Autodesk Inventor part; units mm, degrees
ref_plane "YZ Plane" through (0, 0, 0) normal (1, 0, 0) x (0, 1, 0)
ref_plane "XZ Plane" through (0, 0, 0) normal (0, 1, 0) x (-1, 0, 0)
ref_plane "XY Plane" through (0, 0, 0) normal (0, 0, 1) x (1, 0, 0)
sketch "Sketch1" plane through (0, 0, 0) normal (0, 0, 1) x (1, 0, 0)
  line L0 (-26.797, 26.797) -> (26.797, 26.797)
  line L1 (26.797, 26.797) -> (26.797, -26.797)
  line L2 (26.797, -26.797) -> (-26.797, -26.797)
  line L3 (-26.797, -26.797) -> (-26.797, 26.797)
  point P0 (0, 0)
  point P1 (-26.797, 0)
  point P2 (0, 26.797)
  dimension "d0" = 53.594
  dimension "d1" = 53.594
extrude "Extrusion1" add sketch "Sketch1" along normal blind 38.1
fillet "Fillet1" radius 6.35 2 edges at (-26.797, 26.797, 19.05) (26.797, 26.797, 19.05)
sketch "Sketch3" plane through (0, 0, 38.1) normal (0, 0, 1) x (1, 0, 0)
  arc A0 (26.797, 20.447) -> (20.447, 26.797) centre (20.447, 20.447) ccw
  line L0 (-20.447, 26.797) -> (20.447, 26.797)
  arc A1 (-20.447, 26.797) -> (-26.797, 20.447) centre (-20.447, 20.447) ccw
  line L1 (-26.797, -26.797) -> (-26.797, 20.447)
  line L2 (26.797, -26.797) -> (-26.797, -26.797)
  line L3 (26.797, 20.447) -> (26.797, -26.797)
  arc A2 (-22.5612, -14.4593) -> (-20.447, -26.797) centre (-20.447, -20.447) ccw
  arc A3 (20.447, -26.797) -> (22.5612, -14.4593) centre (20.447, -20.447) ccw
  line L4 (-26.797, -26.797) -> (26.797, -26.797)
  line L5 (-26.797, 0) -> (-26.797, -26.797)
  line L6 (26.797, 0) -> (26.797, -26.797)
  arc A4 (22.5612, -14.4593) -> (-22.5612, -14.4593) centre (0, 0) ccw
  line L7 (-26.797, 0) -> (-26.797, 20.447)
  line L8 (-20.447, 26.797) -> (20.447, 26.797)
  line L9 (26.797, 20.447) -> (26.797, 0)
  arc A5 (-20.447, 26.797) -> (-26.797, 20.447) centre (-20.447, 20.447) ccw
  arc A6 (26.797, 20.447) -> (20.447, 26.797) centre (20.447, 20.447) ccw
  dimension "d9" = 12.7
  dimension "d10" = 12.7
  dimension "d12" = 26.797
extrude "Extrusion2" cut sketch "Sketch3" against normal through all contours L3 A3 A4 | L3 L2 A3 | A4 A2 L1 | A2 L2 L1
fillet "Fillet2" radius 1.5875 2 edges at (22.5612, -14.4593, 19.05) (-22.5612, -14.4593, 19.05)
sketch "Sketch4" plane through (-20.447, 26.797, 0) normal (0, 1, 0) x (1, 0, 0)
  line L0 (0, 0) -> (40.894, 0)
  line L1 (-6.35, -38.1) -> (0, -38.1)
  line L2 (0, -38.1) -> (0, 0)
  line L3 (0, 0) -> (-6.35, 0)
  line L4 (-6.35, 0) -> (-6.35, -38.1)
  line L5 (43.8591, 0) -> (43.8591, -38.1)
  line L6 (40.894, -38.1) -> (47.244, -38.1)
  line L7 (47.244, -38.1) -> (47.244, 0)
  line L8 (47.244, 0) -> (40.894, 0)
  line L9 (40.894, 0) -> (40.894, -38.1)
  line L10 (-2.9651, -38.1) -> (-2.9651, 0)
  circle A0 centre (20.447, -25.4) radius 19.05
  point P0 (20.447, 0)
  point P1 (20.447, -6.35)
  point P2 (20.447, 0)
  dimension "d16" = 38.1
  dimension "d17" = 6.35
extrude "Extrusion3" add sketch "Sketch4" along normal blind 3.175 contours A0
fillet "Fillet3" radius 0.7937 1 edges at (-19.05, 29.972, 25.4)
sketch "Sketch5" plane through (0, 29.972, 25.4) normal (0, 1, 0) x (1, 0, 0)
  circle A0 centre (0, 0) radius 18.2562
  circle A1 centre (0, 0) radius 12.7
  circle A2 centre (0, 0) radius 19.05
  point P0 (0, 25.4)
  dimension "d24" = 6.35
extrude "Extrusion4" add sketch "Sketch5" along normal blind 25.4 contours A1
sketch "Sketch6" plane through (0, 29.972, 25.4) normal (0, 1, 0) x (1, 0, 0)
  circle A0 centre (-14.1881, 8.1915) radius 1.6383
  circle A1 centre (0, -16.383) radius 1.6383
  circle A2 centre (14.1881, 8.1915) radius 1.6383
  point P0 (0, 25.4)
hole "Hole1" at (0, 29.972, 41.783) at (14.1881, 29.972, 17.2085) at (-14.1881, 29.972, 17.2085) direction (0, -1, 0) diameter 3.2766 depth 6.35 tip angle 118
properties part number "Pneumatics_VIAIR_0090_02"
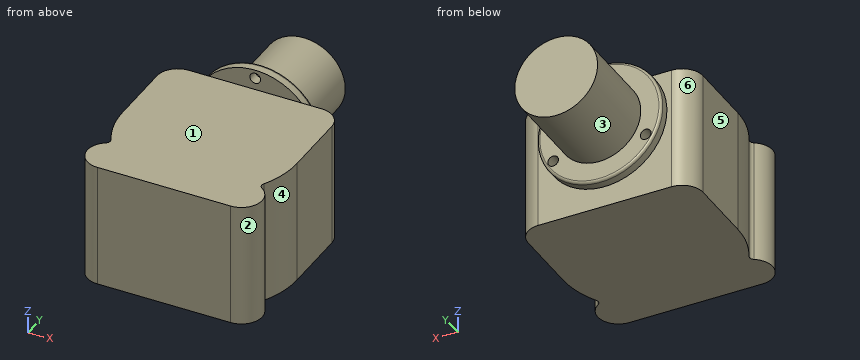
Geometry check sheet. Reference: the model listing, model coordinates, mm. Face numbers are marked on the shaded views. A direction names the side the tool comes from. Round coordinates to 2 decimals unless told otherwise and drop trailing zeros. Order: outer loops, then holes, each group sorted by start corner. A loop starts at its lowest first (then second) coordinate and runs counter-clockwise, first axis right, second up. Notation, with made-up numbers: (-7.5, -36.75) - (43.5, -36.75) arc R28 cw to (43.5, 2.25) - close; hole circle Ø7 at (47, 0). An arc over 180 degrees is marked (long way). One line per question, with ' | ' between items. Start each with the question number.
(1) Sectioned sample at A-A on x = 0. Record the cut outline in (y, z), and give its area (3 significant figures).
(2) Depth check by flat-ended pin: pin 1 Ø2.5 at (x, z) = (14.19, 17.21) entering from +Y; pin 2 Ø3 at (x, y) = (16.5, -7) entering from +Z; pin 3 Ø10 at (y, z) = (38, 36.5) entering from +X. Enter the tip coordinate at first touch or a pass-through.
(3) Sectioned sample at D-D on y = -21. Record the cut outline in (x, z), and give its area (3 significant figures).
(4) Sectioned sample at B-B on y = 35.5. Record the cut outline in (x, z), and give its area (3 significant figures).
(5) Access from +Z, -Z, +X, -X, +Y, -Y to the whole of each face (thin tool, end or side, straight path). Record for the marked faces 1, 2 and 3.
(6) Thickness scan on L1, parallel to Z at x = 0, y = 28.9; L2, parallel to Y at x = -18.5, z = 10.5; L3, parallel to Z at x = -8.5, y = 5.5. Record the ranges inside material, lowest first. Write a range as [from, to].
(7) Sectioned sample at C-C on y = 16.5. Record the cut outline in (x, z).
(8) Release check for a two-part mould opening along Y. For the marked faces 4, 5 and 6 record: released by +Y, released by -Y, zero draft, split by the parting line, or undercut.
Conclusion:
1) outline: (-26.8, 0) - (26.8, 0) - (26.8, 6.35) - (29.18, 6.35) arc R0.79 ccw to (29.97, 7.14) - (29.97, 12.7) - (55.37, 12.7) - (55.37, 38.1) - (29.97, 38.1) - (29.97, 40.14) - (26.8, 40.14) - (26.8, 38.1) - (-26.8, 38.1) - close; (26.8, 43.42) - (29.97, 43.42) - (29.97, 43.66) arc R0.79 ccw to (29.18, 44.45) - (26.8, 44.45) - close | area: 2,800 mm2
2) pin 1: stops at y = 23.39 | pin 2: stops at z = 38.1 | pin 3: stops at x = 11.14
3) outline: (-26.77, 0) - (26.77, 0) - (26.77, 38.1) - (-26.77, 38.1) - close | area: 2,040 mm2
4) outline: circle Ø25.4 at (0, 25.4) | area: 507 mm2
5) face 1: +Z, +X, -X, -Y | face 2: +Z, -Z, +X | face 3: +Y
6) L1: z = [6.35, 40.14], [43.42, 44.45] | L2: y = [-26.8, 26.8] | L3: z = [0, 38.1]
7) outline: (-26.8, 0) - (26.8, 0) - (26.8, 38.1) - (-26.8, 38.1) - close
8) face 4: undercut | face 5: zero draft | face 6: released by +Y
